Work out the finished part from the listing and answer in its coordinate system (mm). A direction names the side the tool comes from. Give positions to 0.01 mm unless a question says otherwise; leave off trailing zeros. Loops run counter-clockwise (first coordinate to the right, second up) from the corner with the lowest first, then second, coordinate; pieces in that order, holes last.
Autodesk Inventor part; units mm, degrees
ref_plane "YZ Plane" through (0, 0, 0) normal (1, 0, 0) x (0, 1, 0)
ref_plane "XZ Plane" through (0, 0, 0) normal (0, 1, 0) x (-1, 0, 0)
ref_plane "XY Plane" through (0, 0, 0) normal (0, 0, 1) x (1, 0, 0)
sketch "スケッチ1" plane through (0, 0, 0) normal (1, 0, 0) x (0, 1, 0)
  arc A0 (45.2642, -8.1944) -> (-45.5834, -6.1769) centre (0, 0) ccw
  arc A1 (-20.1179, -194.1032) -> (11.4813, -194.8049) centre (-4.2628, -191.9547) ccw
  line L0 (45.2642, -8.1944) -> (11.4813, -194.8049)
  line L1 (-45.5834, -6.1769) -> (-20.1179, -194.1032)
  arc A2 (44.2802, -8.0163) -> (-44.5924, -6.0426) centre (0, 0) ccw
  arc A3 (-19.1269, -193.9689) -> (10.4973, -194.6268) centre (-4.2628, -191.9547) ccw
  line L2 (44.2802, -8.0163) -> (10.4973, -194.6268)
  line L3 (-44.5924, -6.0426) -> (-19.1269, -193.9689)
  dimension "d0" = 92
  dimension "d1" = 32
  dimension "d2" = 192.002
  dimension "d3" = 90
extrude "押し出し1" add sketch "スケッチ1" along normal blind 10
properties part number "type5" material "ゴム"
Q1. Section B-B on y = 5.5 is taken. Give the vertices of the cut face in (x, z), plus the area to 3 significant figures.
Q2. Determine the mould class of faces 1 (the face through (10, 30, -90)), 2 (the face through (4.93, 27.625, -100.015)), 3 (the face through (4.93, -33.03, -98.82)) for opening direction Z: +Z half, -Z half, draft (parallel to the pull), parting line (faces both ways), or undercut.
Q3. Consider line 1 along Y through (x, z) = (9.25, -35.5); line 2 along Y through (x, z) = (8, -49); line 3 along Z through (x, y) = (4.5, 8). Determine where each line is inside the solid, lowest interval first.
Q4. Section C-C on z = -189 is taken. Give the vertices of the cut face in (x, y).
Q5. Which of the six approach directions +Z, -Z, +X, -X, +Y, -Y give full straight-line access (tool end or side, diameter ignored) to faces 4 (the face through (4.93, -4.301, -207.955)), 5 (the face through (4.93, -4.299, -206.955))?
Q6. Given pin 1 (5 mm diameter, centred on x = 5, y = 8, fed in from -Z); pin 2 (5 mm diameter, centred on x = 9, y = 16.5, fed in from +Z); pin 3 (2 mm diameter, centred on x = 5, y = -11, fed in from -Z), each flat-ended and moving along its own axis, determine where each tip first touches the part or whether it passes through.
Q7. Section A-A on x = 2.25 is taken. Give the vertices of the cut face in (y, z).
Check result:
1. outline: (0, -204.63) - (10, -204.63) - (10, -203.34) - (0, -203.34) - close; (0, 44.66) - (10, 44.66) - (10, 45.67) - (0, 45.67) - close
1. area: 23.0 mm2
2. face 1: draft
2. face 2: undercut
2. face 3: -Z half
3. line 1: y = -41.61 to -40.6, 39.3 to 40.32
3. line 2: y = -39.78 to -38.77, 36.86 to 37.88
3. line 3: z = -202.23 to -200.59, 44.28 to 45.3
4. outline: (0, -20.81) - (10, -20.81) - (10, -19.8) - (0, -19.8) - close; (0, 11.52) - (10, 11.52) - (10, 12.53) - (0, 12.53) - close
5. face 4: -Z, +X, -X
5. face 5: +X, -X
6. pin 1: stops at z = -204.63
6. pin 2: stops at z = 43.82
6. pin 3: stops at z = -206.89
7. outline: (-45.58, -6.18) - (-20.12, -194.1) arc R16 ccw to (11.48, -194.8) - (45.26, -8.19) arc R46 ccw (long way) to start; hole (-44.59, -6.04) - (-19.13, -193.97) arc R15 ccw to (10.5, -194.63) - (44.28, -8.02) arc R45 ccw (long way) to start
